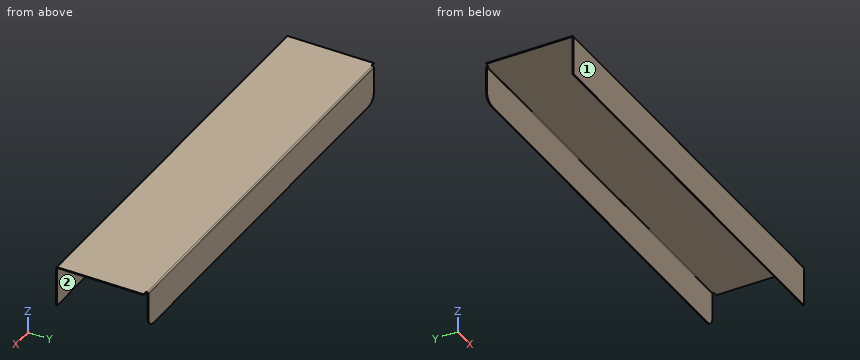
```python
from build123d import *

# Parameters (mm, degrees)
BASE_FLANGE1_DEPTH     = 1
SKETCHED_START         = -232.5
SKETCHED_BEND1_DEPTH   = 465
SKETCHED_START_2       = -227.5
SKETCHED_BEND1_2_DEPTH = 455
SKETCHED_BEND1_3_DEPTH = 465
FILLET1_R              = 10


# Read off the part's stored shape, not the designer's step: Sketched Bend1
# Sheet-metal steps are written as plain solids
with BuildPart() as part:
    # Sketch1 → Base-Flange1 (new body)
    with BuildSketch(Plane.XY):
        Polygon((-227.5, 93), (-227.5, 50), (-232.5, 50), (-232.5, -93), (232.5, -93), (232.5, 50), (227.5, 50), (227.5, 93), align=None)
    extrude(amount=-BASE_FLANGE1_DEPTH)

    # Sketched Bend1 outline → Sketched Bend1 (cut)
    with BuildSketch(Plane.YZ.offset(SKETCHED_START)):
        with BuildLine():
            ThreePointArc((51.028776631, 0), (51.960602795, -0.271171885), (52.601417721, -1))
            Line((52.601417721, -1), (93, -1))
            Line((93, -1), (93, 0))
            Line((93, 0), (51.028776631, 0))
        make_face()
        with BuildLine():
            Line((-93, -1), (-48.601417721, -1))
            ThreePointArc((-48.601417721, -1), (-47.960602795, -0.271171885), (-47.028776631, 0))
            Line((-47.028776631, 0), (-93, 0))
            Line((-93, 0), (-93, -1))
        make_face()
    extrude(amount=SKETCHED_BEND1_DEPTH, mode=Mode.SUBTRACT)

    # Sketched Bend1 2 outline → Sketched Bend1 2 (add)
    with BuildSketch(Plane.YZ.offset(SKETCHED_START_2)):
        with BuildLine():
            ThreePointArc((51.028776631, -1), (51.549631486, -1.215745145), (51.765376631, -1.7366))
            Line((51.765376631, -1.7366), (51.765376631, -41.765376631))
            Line((51.765376631, -41.765376631), (52.765376631, -41.765376631))
            Line((52.765376631, -41.765376631), (52.765376631, -1.7366))
            ThreePointArc((52.765376631, -1.7366), (52.723891388, -1.359286442), (52.601417721, -1))
            Line((52.601417721, -1), (51.028776631, -1))
        make_face()
        with BuildLine():
            ThreePointArc((-47.765376631, -1.7366), (-47.549631486, -1.215745145), (-47.028776631, -1))
            Line((-47.028776631, -1), (-48.601417721, -1))
            ThreePointArc((-48.601417721, -1), (-48.723891388, -1.359286442), (-48.765376631, -1.7366))
            Line((-48.765376631, -1.7366), (-48.765376631, -45.765376631))
            Line((-48.765376631, -45.765376631), (-47.765376631, -45.765376631))
            Line((-47.765376631, -45.765376631), (-47.765376631, -1.7366))
        make_face()
    extrude(amount=SKETCHED_BEND1_2_DEPTH)

    # Sketched Bend1 3 outline → Sketched Bend1 3 (add)
    with BuildSketch(Plane.YZ.offset(SKETCHED_START)):
        with BuildLine():
            ThreePointArc((-47.765376631, -1.7366), (-47.549631486, -1.215745145), (-47.028776631, -1))
            Line((-47.028776631, -1), (-48.601417721, -1))
            ThreePointArc((-48.601417721, -1), (-48.723891388, -1.359286442), (-48.765376631, -1.7366))
            Line((-48.765376631, -1.7366), (-48.765376631, -45.765376631))
            Line((-48.765376631, -45.765376631), (-47.765376631, -45.765376631))
            Line((-47.765376631, -45.765376631), (-47.765376631, -1.7366))
        make_face()
    extrude(amount=SKETCHED_BEND1_3_DEPTH)

    # Fillet1
    fillet1_edges = [part.edges().sort_by_distance(p)[0] for p in [
        (-227.5, 52.265376631, -41.765376631),
        (227.5, 52.265376631, -41.765376631),
    ]]
    fillet(fillet1_edges, radius=FILLET1_R)


solid = part.part
```
Model file for the job. Use its own axes, mm. Face numbers are marked on the shaded views. A direction names the side the tool comes from. Coordinates: 2 decimals unless noted, no trailing zeros. Loops run counter-clockwise (first coordinate to the right, second up) from the corner with the lowest first, then second, coordinate; pieces in that order, holes last. Notation, with made-up numbers: (44.5, 50) - (50.5, 50) arc R26 cw to (50.5, 78) - close; hole circle Ø5 at (65, -37). An arc over 180 degrees is marked (long way). Write item = value, one per line. Start each with the question number.
Item 1: 3-axis set-ups, long thin cutter, end or side, ignore diameter. For the marked faces 1 and 2: which of +Z, -Z, +X, -X, +Y, -Y reach the whole face in a straight line?
Item 2: Drop flat-ended pins along their axis: pin 1 Ø2 at (x, y) = (169, 17.5) entering from -Z; pin 2 Ø12 at (y, z) = (-21.5, -6) entering from -X; pin 3 Ø1.4 at (y, z) = (51, -9) entering from +X; pin 4 Ø0.5 at (x, y) = (105.5, 52.5) entering from -Z. Give the stop position or say it passes through.
Item 3: Saw through at A-A, the plane z = -24. List the corners of the cut face in (x, y).
Item 4: Saw through at C-C, the plane y = 21. List the corners of the cut face in (x, z).
Item 5: Saw through at B-B, the plane x = 105.5. List the corners of the cut face in (y, z).
Item 6: Wall check: probe 1 along Y at (x, z) = (195.5, -9.5); probe 2 along Z at (x, y) = (-66.5, 10). Give the ranges that are in metal, low to high. Write a range as [from, to].
Answers:
q1.face_1 = +Z, -Z, +X, -X, -Y
q1.face_2 = -Z, +X, -X
q2.pin_1 = -1
q2.pin_2 = -232.5
q2.pin_3 = through
q2.pin_4 = -41.77
q3.outline = (-232.5, -48.77) - (232.5, -48.77) - (232.5, -47.77) - (-232.5, -47.77) - close; (-227.5, 51.77) - (227.5, 51.77) - (227.5, 52.77) - (-227.5, 52.77) - close
q4.outline = (-232.5, -1) - (232.5, -1) - (232.5, 0) - (-232.5, 0) - close
q5.outline = (-48.77, -45.77) - (-47.77, -45.77) - (-47.77, -1.74) arc R0.74 cw to (-47.03, -1) - (51.03, -1) arc R0.74 cw to (51.77, -1.74) - (51.77, -41.77) - (52.77, -41.77) - (52.77, -1.74) arc R1.74 ccw to (51.03, 0) - (-47.03, 0) arc R1.74 ccw to (-48.77, -1.74) - close
q6.probe_1 = [-48.77, -47.77], [51.77, 52.77]
q6.probe_2 = [-1, 0]
